```python
from build123d import *

# Parameters (mm, degrees)
F0_R          = 36.999362
F1_DEPTH      = 152.4
F2_R          = 13.360744
F3_DEPTH      = 228.6
F3_DEPTH_BACK = 228.6


with BuildPart() as f1:
    # F0 (on Top) → F1 (new body)
    with BuildSketch(Plane.XY):
        Circle(F0_R)
        Polygon((11.219716, -24.246573), (-15.38829, -21.839846), (-26.608006, 2.406727), (-11.219716, 24.246573), (15.38829, 21.839846), (26.608006, -2.406727), align=None, mode=Mode.SUBTRACT)
    extrude(amount=F1_DEPTH)

    # F2 (on Right) → F3 (cut, two sides)
    with BuildSketch(Plane.YZ) as f3_sk:
        with Locations((0, 75.625911)):
            Circle(F2_R)
    extrude(amount=F3_DEPTH, mode=Mode.SUBTRACT)
    extrude(f3_sk.sketch, amount=-F3_DEPTH_BACK, mode=Mode.SUBTRACT)


solid = f1.part
```
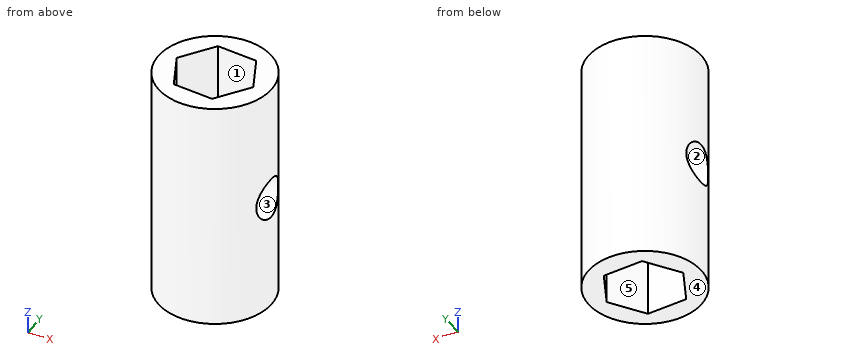
CAD build for the part. Positions are in the model's coordinates, mm. Face numbers are marked on the shaded views. A direction names the side the tool comes from. Give positions to 0.01 mm unless a question says otherwise; leave off trailing zeros. Write each loop counter-clockwise with the first axis right and the second up, starting at its lowest first coordinate (ties: lowest second). Pieces come first, ordered by that corner, then holes. Notation, with made-up numbers: (16, 63.5) -> (49, 63.5) arc R21 cw to (49, 75.5) -> close; hole circle Ø2 at (59, 48.5). An arc over 180 degrees is marked (long way). Write each question's results on one line, items separated by ' | '.
1. Cut at B-B, the plane y = 0. Write the cut outline in (x, z).
Geometry check:
outline: (-37, 0) -> (-25.49, 0) -> (-25.49, 62.27) -> (-37, 62.27) -> close; (-37, 88.99) -> (-25.49, 88.99) -> (-25.49, 152.4) -> (-37, 152.4) -> close; (25.49, 0) -> (37, 0) -> (37, 62.27) -> (25.49, 62.27) -> close; (25.49, 88.99) -> (37, 88.99) -> (37, 152.4) -> (25.49, 152.4) -> close
2. Two-plate mould, pull along Z, no slides. Class the marked faces 3, 4 and 5: pulls with the +Z half, pulls with the -Z half, needs draft (parallel to the pull), parting line crosses it, or undercut.
Geometry check:
face 3: undercut | face 4: pulls with the -Z half | face 5: needs draft
3. Which spindle directions (+Z, -Z, +X, -X, +Y, -Y) get a long thin tool onto all of the face, cutting with end or side? Do the marked faces 1 and 2. Say none if no direction does.
Geometry check:
face 1: +Z, -Z | face 2: +X, -X
4. Wall check: probe 1 along Z at (x, y) = (30.25, 0); probe 2 along Y at (x, z) = (-20, 6.5); probe 3 along Y at (x, z) = (1, 69.5). Give the ranges that are in metal, low to high. Write a range as [from, to].
Geometry check:
probe 1: [0, 62.27], [88.99, 152.4] | probe 2: [-31.13, -11.87], [11.79, 31.13] | probe 3: [-36.99, -23.32], [23.14, 36.99]
5. Cut at C-C, the plane x = 6. Write the cut outline in (y, z).
Geometry check:
outline: (-36.51, 0) -> (-23.77, 0) -> (-23.77, 152.4) -> (-36.51, 152.4) -> close; (22.69, 0) -> (36.51, 0) -> (36.51, 152.4) -> (22.69, 152.4) -> close
6. Cut at D-D, the plane y = 18. Write the cut outline in (x, z).
Geometry check:
outline: (-32.33, 0) -> (-15.62, 0) -> (-15.62, 152.4) -> (-32.33, 152.4) -> close; (17.17, 0) -> (32.33, 0) -> (32.33, 152.4) -> (17.17, 152.4) -> close
7. Drop flat-ended pins along their axis: P1, Ø10, axis at x = -27.5, z = 23, coming from the -Y side; P2, Ø12, axis at y = 28.5, z = 115, coming from the -X side; P3, Ø8, axis at x = 10.5, z = 22, coming from the -Y side. Give the stop position or say it passes through.
Geometry check:
P1: y = -29.37 | P2: x = -29.37 | P3: y = -36.42
8. Cut at A-A, the plane z = 143.5. Write the cut outline in (x, y).
Geometry check:
outline: circle Ø74 at (0, 0); hole (-26.61, 2.41) -> (-15.39, -21.84) -> (11.22, -24.25) -> (26.61, -2.41) -> (15.39, 21.84) -> (-11.22, 24.25) -> close
